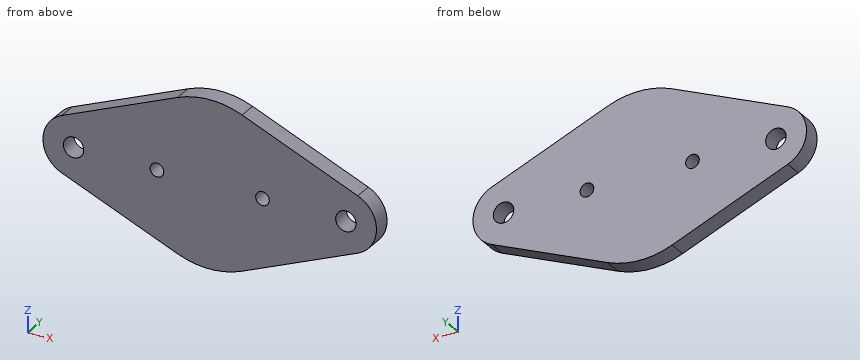
from build123d import *

# Parameters (mm, degrees)
BOSS_EXTRUDE1_DEPTH = 2.7
CUT_EXTRUDE1_REACH  = 4.7
SKETCH2_R           = 1.5
SKETCH2_R_2         = 1


with BuildPart() as part:
    # Sketch1 → Boss-Extrude1 (new body)
    with BuildSketch(Plane(origin=(0, 0, 0), x_dir=(1, 0, 0), z_dir=(0, 1, 0))):
        with BuildLine():
            Line((4.746875, 11.292903866), (21.74375, 4.148413665))
            ThreePointArc((21.74375, 4.148413665), (24.5, 0), (21.74375, -4.148413665))
            Line((21.74375, -4.148413665), (4.746875, -11.292903866))
            ThreePointArc((4.746875, -11.292903866), (0, -12.25), (-4.746875, -11.292903866))
            Line((-4.746875, -11.292903866), (-21.74375, -4.148413665))
            ThreePointArc((-21.74375, -4.148413665), (-24.5, 0), (-21.74375, 4.148413665))
            Line((-21.74375, 4.148413665), (-4.746875, 11.292903866))
            ThreePointArc((-4.746875, 11.292903866), (0, 12.25), (4.746875, 11.292903866))
        make_face()
    extrude(amount=BOSS_EXTRUDE1_DEPTH)

    # Sketch2 → Cut-Extrude1 (cut, up to next)
    with BuildSketch(Plane(origin=(0, 2.7, 0), x_dir=(1, 0, 0), z_dir=(0, 1, 0)), mode=Mode.PRIVATE) as cut_extrude1_sk1:
        with Locations((-20, 0)):
            Circle(SKETCH2_R)
    cut_extrude1_tool1 = extrude(cut_extrude1_sk1.sketch, amount=-CUT_EXTRUDE1_REACH, mode=Mode.PRIVATE) & part.part
    add(cut_extrude1_tool1.solids().sort_by_distance((-20, 2.7, 0))[0], mode=Mode.SUBTRACT)
    # Sketch2 → Cut-Extrude1 (cut, up to next)
    with BuildSketch(Plane(origin=(0, 2.7, 0), x_dir=(1, 0, 0), z_dir=(0, 1, 0)), mode=Mode.PRIVATE) as cut_extrude1_sk2:
        with Locations((20, 0)):
            Circle(SKETCH2_R)
    cut_extrude1_tool2 = extrude(cut_extrude1_sk2.sketch, amount=-CUT_EXTRUDE1_REACH, mode=Mode.PRIVATE) & part.part
    add(cut_extrude1_tool2.solids().sort_by_distance((20, 2.7, 0))[0], mode=Mode.SUBTRACT)
    # Sketch2 → Cut-Extrude1 (cut, up to next)
    with BuildSketch(Plane(origin=(0, 2.7, 0), x_dir=(1, 0, 0), z_dir=(0, 1, 0)), mode=Mode.PRIVATE) as cut_extrude1_sk3:
        with Locations((7.75, 0)):
            Circle(SKETCH2_R_2)
    cut_extrude1_tool3 = extrude(cut_extrude1_sk3.sketch, amount=-CUT_EXTRUDE1_REACH, mode=Mode.PRIVATE) & part.part
    add(cut_extrude1_tool3.solids().sort_by_distance((7.75, 2.7, 0))[0], mode=Mode.SUBTRACT)
    # Sketch2 → Cut-Extrude1 (cut, up to next)
    with BuildSketch(Plane(origin=(0, 2.7, 0), x_dir=(1, 0, 0), z_dir=(0, 1, 0)), mode=Mode.PRIVATE) as cut_extrude1_sk4:
        with Locations((-7.75, 0)):
            Circle(SKETCH2_R_2)
    cut_extrude1_tool4 = extrude(cut_extrude1_sk4.sketch, amount=-CUT_EXTRUDE1_REACH, mode=Mode.PRIVATE) & part.part
    add(cut_extrude1_tool4.solids().sort_by_distance((-7.75, 2.7, 0))[0], mode=Mode.SUBTRACT)


solid = part.part
The listing builds one solid part. Answer for the finished solid, in the listing's coordinates (mm). Give positions to 0.01 mm unless a question says otherwise; leave off trailing zeros. Loops run counter-clockwise (first coordinate to the right, second up) from the corner with the lowest first, then second, coordinate; pieces in that order, holes last. Notation, with made-up numbers: (-10.5, 4.25) - (43.5, 4.25) arc R14 ccw to (43.5, 19.25) - close; hole circle Ø8 at (69, 0.25). An arc over 180 degrees is marked (long way). Write each question's results on one line, items separated by ' | '.
1. Find section C-C, the plane x = -20. Write down the section's boundary in (y, z).
Resolved:
outline: (0, -4.88) - (2.7, -4.88) - (2.7, -1.5) - (0, -1.5) - close; (0, 1.5) - (2.7, 1.5) - (2.7, 4.88) - (0, 4.88) - close
2. Flat-ended cylindrical pins translate along their axes: P1, Ø4, axis at x = 4.5, z = 1.5, coming from the -Y side; P2, Ø1.5, axis at x = -6.5, y = 2, coming from the +Z side. Find the tip coordinate at first contact, or state that the pin passes through.
Resolved:
P1: stops at y = 0 | P2: stops at z = 10.87
3. Find section D-D, the plane x = -7.75. Write down the section's boundary in (y, z), then the cut area to 3 significant figures.
Resolved:
outline: (0, -10.03) - (2.7, -10.03) - (2.7, -1) - (0, -1) - close; (0, 1) - (2.7, 1) - (2.7, 10.03) - (0, 10.03) - close | area: 48.8 mm^2
4. Find section A-A, the plane z = 0. Write down the section's boundary in (x, y), then the cut area to 3 significant figures.
Resolved:
outline: (-24.5, 0) - (-21.5, 0) - (-21.5, 2.7) - (-24.5, 2.7) - close; (-18.5, 0) - (-8.75, 0) - (-8.75, 2.7) - (-18.5, 2.7) - close; (-6.75, 0) - (6.75, 0) - (6.75, 2.7) - (-6.75, 2.7) - close; (8.75, 0) - (18.5, 0) - (18.5, 2.7) - (8.75, 2.7) - close; (21.5, 0) - (24.5, 0) - (24.5, 2.7) - (21.5, 2.7) - close | area: 105 mm^2
5. Find section B-B, the plane y = 0.75. Write down the section's boundary in (x, z).
Resolved:
outline: (-21.74, -4.15) - (-4.75, -11.29) arc R12.25 ccw to (4.75, -11.29) - (21.74, -4.15) arc R4.5 ccw to (21.74, 4.15) - (4.75, 11.29) arc R12.25 ccw to (-4.75, 11.29) - (-21.74, 4.15) arc R4.5 ccw to start; hole circle Ø3 at (-20, 0); hole circle Ø2 at (-7.75, 0); hole circle Ø2 at (7.75, 0); hole circle Ø3 at (20, 0)
6. Consider probe 1 along Z at (x, y) = (-7.75, 1.9); probe 2 along Z at (x, y) = (-20, 1.05); probe 3 along X at (y, z) = (2.25, -8.5). Determine where each line is inside the solid, lowest interval first. Write a range as from..to.
Resolved:
probe 1: z = -10.03..-1, 1..10.03 | probe 2: z = -4.88..-1.5, 1.5..4.88 | probe 3: x = -11.39..11.39
